```python
from build123d import *

# Parameters (mm, degrees)
BOSS_EXTRUDE1_DEPTH = 98
SKETCH2_W           = 7
SKETCH2_H           = 16
SKETCH2_W_2         = 13.165812667
SKETCH2_H_2         = 15.5
CUT_EXTRUDE1_DEPTH  = 108.088748242
SKETCH4_W           = 12.746406598
SKETCH4_H           = 11.424724901
CUT_EXTRUDE3_DEPTH  = 5
SKETCH5_W           = 15.019607204
SKETCH5_H           = 11.204049301
CUT_EXTRUDE4_DEPTH  = 5
SKETCH6_W           = 13.795170111
SKETCH6_H           = 11.126039216
CUT_EXTRUDE5_DEPTH  = 5
SKETCH7_W           = 13.688711878
SKETCH7_H           = 12.195602477
CUT_EXTRUDE6_DEPTH  = 5


with BuildPart() as part:
    # Sketch1 → Boss-Extrude1 (new body)
    with BuildSketch(Plane.XY):
        with BuildLine():
            Line((0, 0), (30, 0))
            Line((30, 0), (32, 0))
            Line((32, 0), (37, 0))
            ThreePointArc((37, 0), (39.236067977, 9.472135955), (33, 2))
            Line((33, 2), (35.197224362, 2))
            ThreePointArc((35.197224362, 2), (37.935414347, 8.372684391), (37, 1.5))
            Line((37, 1.5), (32, 1.5))
            Line((32, 1.5), (30, 1.5))
            Line((30, 1.5), (0, 1.5))
            Line((0, 1.5), (0, 0))
        make_face()
    extrude(amount=BOSS_EXTRUDE1_DEPTH)

    # Sketch2 → Cut-Extrude1 (cut, through all)
    with BuildSketch(Plane.XZ):
        with Locations((33.5, 49)):
            Rectangle(SKETCH2_W, SKETCH2_H)
        with Locations((43.582906334, 49)):
            Rectangle(SKETCH2_W_2, SKETCH2_H)
        with Locations((33.5, 7.75)):
            Rectangle(SKETCH2_W, SKETCH2_H_2)
        with Locations((43.582906334, 7.75)):
            Rectangle(SKETCH2_W_2, SKETCH2_H_2)
        with Locations((33.5, 90.25)):
            Rectangle(SKETCH2_W, SKETCH2_H_2)
        with Locations((43.582906334, 90.25)):
            Rectangle(SKETCH2_W_2, SKETCH2_H_2)
    extrude(amount=-CUT_EXTRUDE1_DEPTH, mode=Mode.SUBTRACT)

    # Sketch4 → Cut-Extrude3 (cut)
    with BuildSketch(Plane.XY.offset(82.5)):
        with Locations((36.373203299, 5.712362451)):
            Rectangle(SKETCH4_W, SKETCH4_H)
    extrude(amount=-CUT_EXTRUDE3_DEPTH, mode=Mode.SUBTRACT)

    # Sketch5 → Cut-Extrude4 (cut)
    with BuildSketch(Plane(origin=(0, 0, 57), x_dir=(-1, 0, 0), z_dir=(0, 0, -1))):
        with Locations((-37.509803602, 5.602024651)):
            Rectangle(SKETCH5_W, SKETCH5_H)
    extrude(amount=-CUT_EXTRUDE4_DEPTH, mode=Mode.SUBTRACT)

    # Sketch6 → Cut-Extrude5 (cut)
    with BuildSketch(Plane.XY.offset(41)):
        with Locations((36.897585056, 5.563019608)):
            Rectangle(SKETCH6_W, SKETCH6_H)
    extrude(amount=-CUT_EXTRUDE5_DEPTH, mode=Mode.SUBTRACT)

    # Sketch7 → Cut-Extrude6 (cut)
    with BuildSketch(Plane(origin=(0, 0, 15.5), x_dir=(-1, 0, 0), z_dir=(0, 0, -1))):
        with Locations((-36.844355939, 6.097801239)):
            Rectangle(SKETCH7_W, SKETCH7_H)
    extrude(amount=-CUT_EXTRUDE6_DEPTH, mode=Mode.SUBTRACT)


solid = part.part
```
Geometry: final body of the model. Coordinates: model frame, mm. A direction names the side the tool comes from. Give positions to 0.01 mm unless a question says otherwise; leave off trailing zeros. Write each loop counter-clockwise with the first axis right and the second up, starting at its lowest first coordinate (ties: lowest second). Pieces come first, ordered by that corner, then holes.
1. Section query D-D, the plane x = 18.5. Return loops of the section in (y, z), then the cut area to 3 significant figures.
2. Section query C-C, the plane x = 39. Return loops of the section in (y, z).
3. Draft query along Y for faces 1 (the flat face through (34, 2, 70)), 2 (the flat face through (14, 0, 48)), 3 (the flat face through (34, 2, 28)), 4 (the flat face through (33, 5, 20.5)). Return one class per face: released by +Y, released by -Y, zero draft, split by the parting line, or undercut.
4. Line query: probe 1 along X at (y, z) = (5, 66.5); probe 2 along Y at (x, z) = (37, 24.5); probe 3 along Y at (x, z) = (27.5, 87.5). Output: solid intervals per line, ascending.
5. Section query B-B, the plane z = 63. Return loops of the section in (x, y), then the cut area to 3 significant figures.
6. Reachability of faces 5 (the flat face through (33.7, 3.2, 77.5)), 6 (the cylindrical face through (37.799, 8.408, 28.142)), 7 (the flat face through (33.7, 3.2, 36)) from +Z, -Z, +X, -X, +Y, -Y: full face, straight path, thin tool, end or side. Return the list, or none.
7. Section query A-A, the plane y = 5. Return loops of the section in (x, z), then the cut area to 3 significant figures.
8. Pin query (flat end, axial travel): P1, Ø1.2, axis at y = 0.5, z = 46, coming from the +X side; P2, Ø1, axis at y = 2.5, z = 54, coming from the +X side (1 decimal); P3, Ø8, axis at x = 20, z = 40.5, coming from the +Y side. Return the tip coordinate at first contact, or that it passes through.
Computed:
1. outline: (0, 0) - (1.5, 0) - (1.5, 98) - (0, 98) - close
1. area: 147 mm2
2. outline: (0.42, 20.5) - (2.13, 20.5) - (2.13, 36) - (0.42, 36) - close; (0.42, 62) - (2.13, 62) - (2.13, 77.5) - (0.42, 77.5) - close; (7.87, 20.5) - (9.58, 20.5) - (9.58, 36) - (7.87, 36) - close; (7.87, 62) - (9.58, 62) - (9.58, 77.5) - (7.87, 77.5) - close
3. face 1: undercut
3. face 2: released by -Y
3. face 3: undercut
3. face 4: zero draft
4. probe 1: x = 32 to 33.5, 40.5 to 42
4. probe 2: y = 0 to 1.5, 8.5 to 10
4. probe 3: y = 0 to 1.5
5. outline: (0, 0) - (37, 0) arc R5 ccw (long way) to (33, 2) - (35.2, 2) arc R3.5 cw (long way) to (37, 1.5) - (0, 1.5) - close
5. area: 90.6 mm2
6. face 5: +Z, +X, +Y, -Y
6. face 6: +Z, -Z
6. face 7: +X, +Y, -Y
7. outline: (32, 20.5) - (33.5, 20.5) - (33.5, 36) - (32, 36) - close; (32, 62) - (33.5, 62) - (33.5, 77.5) - (32, 77.5) - close; (40.5, 20.5) - (42, 20.5) - (42, 36) - (40.5, 36) - close; (40.5, 62) - (42, 62) - (42, 77.5) - (40.5, 77.5) - close
7. area: 93.0 mm2
8. P1: stops at x = 30
8. P2: passes through
8. P3: stops at y = 1.5
